Check sheet for the modelled part. Datum: model origin and axes. Units: mm. A direction names the side the tool comes from. Give positions to 0.01 mm unless a question says otherwise; leave off trailing zeros. Order: outer loops, then holes, each group sorted by start corner. A loop starts at its lowest first (then second) coordinate and runs counter-clockwise, first axis right, second up.
Item 1: Access from +Z, -Z, +X, -X, +Y, -Y to the whole of each face (thin tool, end or side, straight path). Record for faces 1 (the flat face through (-102, -18.459, 22)), 2 (the flat face through (-102, -13, 16.852)), 3 (the flat face through (-102, -8.613, 22)), 4 (the flat face through (-102, -13, 26.638)).
Item 2: Sectioned sample at B-B on y = -6.5. Record the boundary of the cut face in (x, z), and give its area (3 significant figures).
Item 3: Material ranges on line 1 along Y through (x, z) = (-119, 22.5); line 2 along Z through (x, y) = (-73.5, -15.75); line 3 along X through (y, z) = (-12.75, 16.75), recorded low to high.
Item 4: Gauge pin test, flat ends, axial feed: P1, Ø8, axis at y = -3, z = 25, coming from the -X side; P2, Ø11, axis at x = -107.5, z = 23, coming from the +Y side; P3, Ø3, axis at x = -90, y = -14.5, coming from the +Z side. Record the tip position at first contact, or that the pin passes through.
Item 5: Sectioned sample at C-C on x = -126. Record the boundary of the cut face in (y, z).
Item 6: Sectioned sample at A-A on z = 23. Record the boundary of the cut face in (x, y).
from build123d import *

# Parameters (mm, degrees)
F0_W     = 50.8
F0_H     = 27.1318203053
F1_DEPTH = 25.4
F2_DEPTH = 25.4
F4_W     = 9.8461210728
F4_H     = 9.7858998924
F5_DEPTH = 62.9539089


# Not quite as in the source:
# - an extrude ends at something that could not be found from the text; its depth is read off the source's solid


with BuildPart() as f1:
    # F0 (on Front) → F1 (new body)
    with BuildSketch(Plane.XZ):
        with Locations((-45.1160669327, 19.4199038669)):
            Rectangle(F0_W, F0_H)
    extrude(amount=F1_DEPTH)

    # F2 (add): a face of the model
    f2_faces = [f1.faces().sort_by_distance(p)[0] for p in [
        (-70.5160669327, -12.7, 19.4199038669),
    ]]
    extrude(f2_faces, amount=-F2_DEPTH)

    # F4 (on face) → F5 (join, through all)
    with BuildSketch(Plane(origin=(-70.5160669327, 0, 0), x_dir=(0, -1, 0), z_dir=(-1, 0, 0))):
        with Locations((13.5363917798, 21.7452598736)):
            Rectangle(F4_W, F4_H)
    extrude(amount=F5_DEPTH)


solid = f1.part
Report:
1. face 1: +Z, -Z, -X, -Y
1. face 2: -Z, -X, +Y, -Y
1. face 3: +Z, -Z, -X, +Y
1. face 4: +Z, -X, +Y, -Y
2. outline: (-70.52, 5.85) - (-19.72, 5.85) - (-19.72, 32.99) - (-70.52, 32.99) - close
2. area: 1,380 mm2
3. line 1: y = -18.46 to -8.61
3. line 2: z = 16.85 to 26.64
3. line 3: x = -70.52 to -19.72
4. P1: stops at x = -70.52
4. P2: stops at y = -8.61
4. P3: stops at z = 26.64
5. outline: (-18.46, 16.85) - (-8.61, 16.85) - (-8.61, 26.64) - (-18.46, 26.64) - close
6. outline: (-133.47, -18.46) - (-70.52, -18.46) - (-70.52, -25.4) - (-19.72, -25.4) - (-19.72, 0) - (-70.52, 0) - (-70.52, -8.61) - (-133.47, -8.61) - close
